Geometry check sheet. Reference: the model listing, model coordinates, mm. Round coordinates to 2 decimals unless told otherwise and drop trailing zeros. Write each loop counter-clockwise with the first axis right and the second up, starting at its lowest first coordinate (ties: lowest second). Pieces come first, ordered by that corner, then holes. Notation, with made-up numbers: (81.25, 41) - (131.25, 41) arc R13 cw to (131.25, 49) - close; hole circle Ø10 at (43, 31.25). An arc over 180 degrees is marked (long way). Return JSON: item names as keys, results as strings.
```python
from build123d import *

# Parameters (mm, degrees)
ESQUISSE1_W             = 40
ESQUISSE1_H             = 35
ESQUISSE1_W_2           = 12
ESQUISSE1_H_2           = 2.5
BOSS_EXTRU_1_DEPTH      = 2
ENL_V_MAT_EXTRU_1_DEPTH = 10


with BuildPart() as part:
    # Esquisse1 → Boss.-Extru.1 (new body)
    with BuildSketch(Plane(origin=(0, 0, 0), x_dir=(1, 0, 0), z_dir=(0, 1, 0))):
        Rectangle(ESQUISSE1_W, ESQUISSE1_H)
        with BuildLine():
            Line((6.15, 1.220085228), (6.15, 0))
            ThreePointArc((6.15, 0), (9, -2.85), (11.85, 0))
            Line((11.85, 0), (11.85, 1.220085228))
            ThreePointArc((11.85, 1.220085228), (9, 12.5), (6.15, 1.220085228))
        make_face(mode=Mode.SUBTRACT)
        with Locations((-9, -11.25)):
            Rectangle(ESQUISSE1_W_2, ESQUISSE1_H_2, mode=Mode.SUBTRACT)
    extrude(amount=BOSS_EXTRU_1_DEPTH)

    # Esquisse2 → Enlèv. mat.-Extru.1 (cut)
    with BuildSketch(Plane(origin=(0, 2, 0), x_dir=(1, 0, 0), z_dir=(0, 1, 0))):
        with BuildLine():
            Line((-28.745227889, -17.5), (-25.633077883, 26.552925175))
            Line((-25.633077883, 26.552925175), (4.116600537, 17.5))
            add(Edge.make_bspline(
                [(4.116600537, 17.5), (-20.262864911, 6.720677368), (-28.745227889, -17.5)],
                knots=[0, 0, 0, 1, 1, 1], degree=2))
        make_face()
    extrude(amount=-ENL_V_MAT_EXTRU_1_DEPTH, mode=Mode.SUBTRACT)


solid = part.part
```
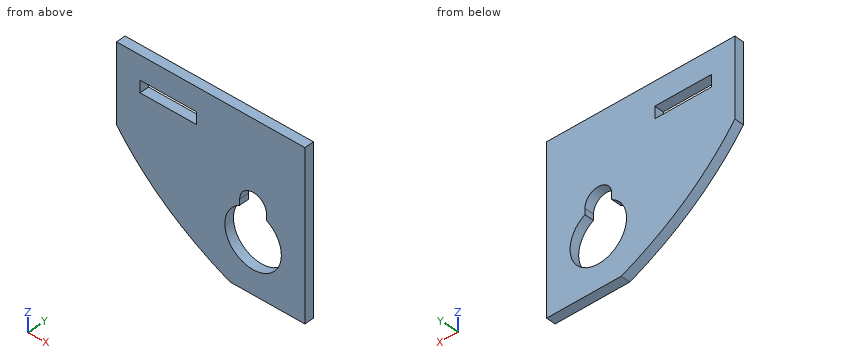
(1) Section check B-B, the plane y = 0.95. Give the number of separate pieces and of enclosed holes in the cut face, plus the area to 3 significant figures.
Response values:
{"separate pieces": "1", "enclosed holes": "2", "area": "1,060 mm^2"}
(2) Section check A-A, the plane x = 9. Enter the section's corners in (y, z).
Response values:
{"outline": "(0, -17.5) - (2, -17.5) - (2, -12.5) - (0, -12.5) - close; (0, 2.85) - (2, 2.85) - (2, 17.5) - (0, 17.5) - close"}
(3) Material ranges on line 1 along Z through (x, y) = (9, 1.1); line 2 along X through (y, z) = (0.25, 12); line 3 along X through (y, z) = (1.5, -6.5), recorded low to high. Write a range as [from, to].
Response values:
{"line 1": "z = [-17.5, -12.5], [2.85, 17.5]", "line 2": "x = [-20, -15], [-3, 20]", "line 3": "x = [-13.09, 3], [15, 20]"}
(4) Gauge pin test, flat end, axial feed: pin 1 (4 mm diameter, centred on x = -6.5, z = -1, fed in from -Y). Record the tip position at first contact, or that the pin passes through.
Response values:
{"pin 1": "stops at y = 0"}
